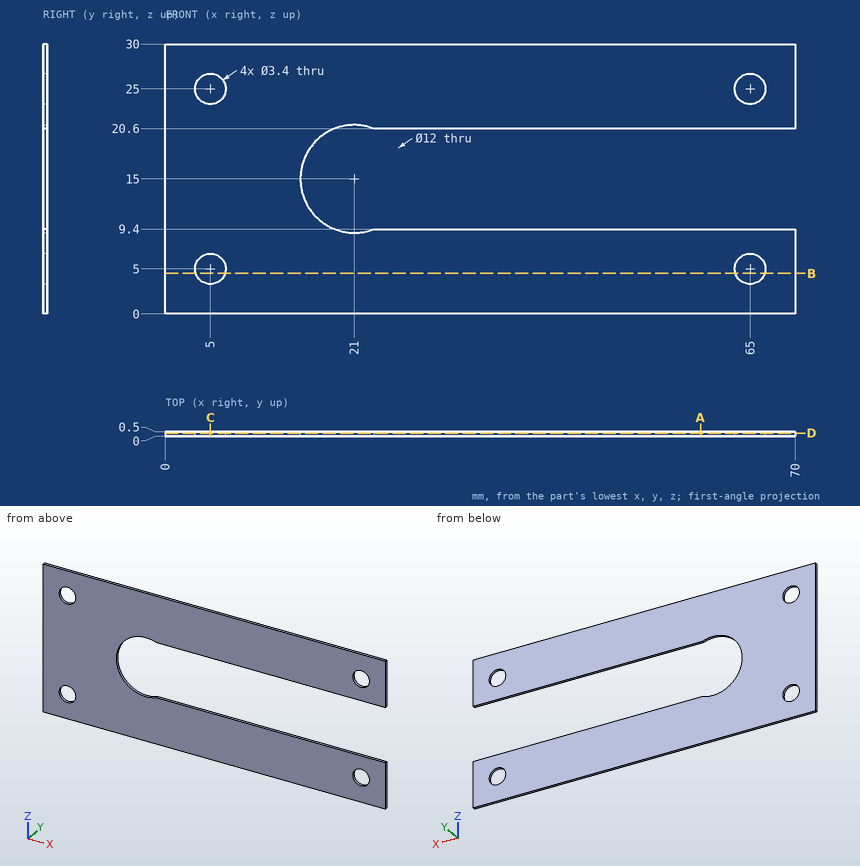
For this review, use the dimensioned drawing (mm, ordinates from the lowest corner) and the shaded views. Coordinates: 2 decimals unless noted, no trailing zeros. Loops run counter-clockwise (first coordinate to the right, second up) from the corner with the lowest first, then second, coordinate; pieces in that order, holes last. Notation, with made-up numbers: M 36.5,83.5 L 51.5,83.5 A30 cw 51.5,108.5 Z; hole C 10,-29.5 d10. An arc over 180 degrees is marked long. Answer as CSV lines item,"result".
Item 1: For probe 1 along X at (y, z) = (0.15, 25); probe 2 along Z at (x, y) = (65, 0.35); probe 3 along X at (y, z) = (0.35, 4.5), list the stretches that pass through material, from the lowest coordinate up.
Answer list:
probe 1,"0 to 3.3, 6.7 to 63.3, 66.7 to 70"
probe 2,"0 to 3.3, 6.7 to 9.4, 20.6 to 23.3, 26.7 to 30"
probe 3,"0 to 3.38, 6.62 to 63.38, 66.62 to 70"
Item 2: Add section C-C on x = 5. State the section outline as (y, z) points.
Answer list:
outline,"M 0,0 L 0.5,0 L 0.5,3.3 L 0,3.3 Z; M 0,6.7 L 0.5,6.7 L 0.5,23.3 L 0,23.3 Z; M 0,26.7 L 0.5,26.7 L 0.5,30 L 0,30 Z"
Item 3: Add section B-B on z = 4.5. State the section outline as (x, y) points.
Answer list:
outline,"M 0,0 L 3.38,0 L 3.38,0.5 L 0,0.5 Z; M 6.62,0 L 63.38,0 L 63.38,0.5 L 6.62,0.5 Z; M 66.62,0 L 70,0 L 70,0.5 L 66.62,0.5 Z"
Item 4: Add section D-D on y = 0.35. State the section outline as (x, z) points, plus the area to 3 significant figures.
Answer list:
outline,"M 0,0 L 70,0 L 70,9.4 L 23.15,9.4 A6 cw long 23.15,20.6 L 70,20.6 L 70,30 L 0,30 Z; hole C 5,5 d3.4; hole C 5,25 d3.4; hole C 65,5 d3.4; hole C 65,25 d3.4"
area,"1,460 mm²"
Item 5: Add section A-A on x = 59.5. State the section outline as (y, z) points.
Answer list:
outline,"M 0,0 L 0.5,0 L 0.5,9.4 L 0,9.4 Z; M 0,20.6 L 0.5,20.6 L 0.5,30 L 0,30 Z"
